The listing builds one solid part. Answer for the finished solid, in the listing's coordinates (mm). A direction names the side the tool comes from. Round coordinates to 2 decimals unless told otherwise and drop trailing zeros. Loops run counter-clockwise (first coordinate to the right, second up) from the corner with the lowest first, then second, coordinate; pieces in that order, holes last. Notation, with made-up numbers: (-35, 55) -> (-15, 55) arc R30 ccw to (-15, 90) -> close; hole circle Ø7 at (32.25, 89.25). An arc over 180 degrees is marked (long way). One line per question, with ' | ' between items.
from build123d import *

# Parameters (mm, degrees)
F0_R     = 24.5
F0_R_2   = 3
F1_DEPTH = 16
F2_W     = 26.459999
F2_H     = 9.765
F3_DEPTH = 25


with BuildPart() as f1:
    # F0 (on Front) → F1 (new body)
    with BuildSketch(Plane.XZ):
        Circle(F0_R)
        Circle(F0_R_2, mode=Mode.SUBTRACT)
    extrude(amount=F1_DEPTH)

    # F2 (on Front) → F3 (cut)
    with BuildSketch(Plane.XZ):
        Polygon((7.513219, 2.936858), (20.743218, 25.851889), (12.28648, 30.734389), (-0.943519, 7.819358), align=None)
        Polygon((-1.213216, -7.975067), (12.016783, -30.890099), (20.473521, -26.007599), (7.243522, -3.092567), align=None)
        with Locations((-19.530002, 0.15571)):
            Rectangle(F2_W, F2_H)
    extrude(amount=F3_DEPTH, mode=Mode.SUBTRACT)


solid = f1.part
Q1. Given pin 1 Ø8 at (x, y) = (-11.5, -14) entering from -Z; pin 2 Ø3 at (y, z) = (-10, 2) entering from -X; pin 3 Ø5 at (y, z) = (-7.5, -11) entering from -X; pin 4 Ø4 at (x, z) = (-19, -19) entering from +Y, each flat-ended and moving along its own axis, determine where each tip first touches the part or whether it passes through.
Numbers:
pin 1: z = -23.32 | pin 2: x = -6.3 | pin 3: x = -22.98 | pin 4: through
Q2. A cutting plane is placed at A-A on z = 0. Give the vertices of the cut face in (x, y).
Numbers:
outline: (-6.3, -16) -> (-3, -16) -> (-3, 0) -> (-6.3, 0) -> close; (3, -16) -> (24.5, -16) -> (24.5, 0) -> (3, 0) -> close
Q3. For a pull along Z with two mould halves and no side action, classify faces 4 (the face through (24.496, -7.888, -0.449)), 5 (the face through (-6, -16, 0)), 6 (the face through (-12.637, -7.888, -20.989)), 7 (the face through (3.553, -7.888, 15.608)) as pulls with the +Z half, pulls with the -Z half, needs draft (parallel to the pull), parting line crosses it, or undercut.
Numbers:
face 4: parting line crosses it | face 5: needs draft | face 6: pulls with the -Z half | face 7: undercut
Q4. A cutting plane is placed at D-D on x = 6. Give the vertices of the cut face in (y, z).
Numbers:
outline: (-16, -23.75) -> (0, -23.75) -> (0, -20.47) -> (-16, -20.47) -> close; (-16, -3.81) -> (0, -3.81) -> (0, 3.81) -> (-16, 3.81) -> close; (-16, 19.85) -> (0, 19.85) -> (0, 23.75) -> (-16, 23.75) -> close
Q5. A cutting plane is placed at B-B on y = -11.25. Give the vertices of the cut face in (x, z).
Numbers:
outline: (-24.04, -4.73) arc R24.5 ccw to (7.62, -23.28) -> (-1.21, -7.98) -> (7.24, -3.09) -> (16.11, -18.46) arc R24.5 ccw to (16.35, 18.25) -> (7.51, 2.94) -> (-0.94, 7.82) -> (7.93, 23.18) arc R24.5 ccw to (-23.98, 5.04) -> (-6.3, 5.04) -> (-6.3, -4.73) -> close; hole circle Ø6 at (0, 0)
Q6. For faces 1 (the face through (-6.3, -8, 0)), 2 (the face through (3.144, -7.888, -15.522)), 3 (the face through (-11.86, -7.89, 21.44)), determine the directions among +Z, -Z, +X, -X, +Y, -Y from which every point of the face is accessible in a straight line to the end or side of a thin tool.
Numbers:
face 1: -X, +Y, -Y | face 2: +Y, -Y | face 3: +Z, +Y, -Y
Q7. Find the intervals of material crossed by line 1 (Z direction, x = 0, y = -3.5); line 2 (Z direction, x = 1, y = -14.5); line 3 (Z direction, x = -17.5, y = -10.25), in increasing order. Write a range as from..to.
Numbers:
line 1: -24.5..-10.08, -7.27..-3, 3..7.27, 9.45..24.5 | line 2: -24.48..-11.81, -6.7..-2.83, 2.83..6.7, 11.19..24.48 | line 3: -17.15..-4.73, 5.04..17.15
Q8. A cutting plane is placed at C-C on x = 0. Give the vertices of the cut face in (y, z).
Numbers:
outline: (-16, -24.5) -> (0, -24.5) -> (0, -10.08) -> (-16, -10.08) -> close; (-16, -7.27) -> (0, -7.27) -> (0, -3) -> (-16, -3) -> close; (-16, 3) -> (0, 3) -> (0, 7.27) -> (-16, 7.27) -> close; (-16, 9.45) -> (0, 9.45) -> (0, 24.5) -> (-16, 24.5) -> close
